For this review, take the finished solid that the model builds, in its own axes (mm). Face numbers are marked on the shaded views. A direction names the side the tool comes from. Coordinates: 2 decimals unless noted, no trailing zeros. Write each loop counter-clockwise with the first axis right and the second up, starting at its lowest first coordinate (ties: lowest second). Pieces come first, ordered by that corner, then holes. Notation, with made-up numbers: (32.25, 77.25) -> (45.25, 77.25) arc R19 ccw to (45.25, 81.25) -> close; hole circle Ø6 at (69.25, -4.5). An arc over 180 degrees is marked (long way). One line per item, written item: value. Start each with the question number.
1) Add section C-C (x = 8.75). State the section outline as (y, z) points.
2) Add section D-D (x = 4.5). State the section outline as (y, z) points, and give its area (3 significant figures).
3) For pin 1 Ø1.5 at (x, y) = (12.5, 31.5) entering from +Z; pin 2 Ø5.5 at (x, z) = (11.5, -1.5) entering from +Y; pin 3 Ø1 at (x, y) = (15, 2) entering from -Z, all flat-tipped, find the tip position at first contact; note any pin that passes through.
4) Add section A-A (x = 17.5). State the section outline as (y, z) points, and give its area (3 significant figures).
5) For probe 1 along Y at (x, z) = (10, -32.75); probe 2 along X at (y, z) = (34, -2.5); probe 3 along Y at (x, z) = (10.75, -31), list the stretches that pass through material, from the lowest coordinate up. Write a range as from..to.
6) Add section B-B (y = 4.5). State the section outline as (x, z) points.
7) Machinability: for the marked faces 1, 2 and 3, which of the approach directions +Z, -Z, +X, -X, +Y, -Y give a long, thin tool a straight path to every point of the face, cutting with its end or side? Answer none if there is none.
from build123d import *

# Parameters (mm, degrees)
SKETCH1_W           = 20
SKETCH1_H           = 46
BOSS_EXTRUDE1_DEPTH = 35
SKETCH2_W           = 5
SKETCH2_H           = 8
CUT_EXTRUDE1_DEPTH  = 5
FILLET1_R           = 2.5
FILLET2_R           = 1
FILLET3_R           = 1
SKETCH3_R           = 9
SKETCH3_R_2         = 6.5
CUT_EXTRUDE2_DEPTH  = 5
FILLET4_R           = 2
FILLET5_R           = 1


with BuildPart() as part:
    # Sketch1 → Boss-Extrude1 (new body)
    with BuildSketch(Plane.XY):
        with Locations((10, 23)):
            Rectangle(SKETCH1_W, SKETCH1_H)
    extrude(amount=-BOSS_EXTRUDE1_DEPTH)

    # Sketch2 → Cut-Extrude1 (cut)
    with BuildSketch(Plane.XY):
        Polygon((10, 41), (2, 41), (2, 46), (20, 46), (20, 41), align=None)
        with Locations((12.5, 32)):
            Rectangle(SKETCH2_W, SKETCH2_H)
    extrude(amount=-CUT_EXTRUDE1_DEPTH, mode=Mode.SUBTRACT)

    # Fillet1
    fillet1_edges = [part.edges().sort_by_distance(p)[0] for p in [
        (11, 41, -5),
    ]]
    fillet(fillet1_edges, radius=FILLET1_R)

    # Fillet2
    fillet2_edges = [part.edges().sort_by_distance(p)[0] for p in [
        (1, 46, 0),
    ]]
    fillet(fillet2_edges, radius=FILLET2_R)

    # Fillet3
    fillet3_edges = [part.edges().sort_by_distance(p)[0] for p in [
        (11, 46, -5),
        (11, 41, 0),
    ]]
    fillet(fillet3_edges, radius=FILLET3_R)

    # Sketch3 → Cut-Extrude2 (cut)
    with BuildSketch(Plane(origin=(0, 0, -35), x_dir=(-1, 0, 0), z_dir=(0, 0, -1))):
        with Locations((-10, 36)):
            Circle(SKETCH3_R)
        with Locations((-10, 36)):
            Circle(SKETCH3_R_2, mode=Mode.SUBTRACT)
        Polygon((-10, 5), (-20, 5), (-20, 0), (-5, 0), (-5, 5), align=None)
    extrude(amount=-CUT_EXTRUDE2_DEPTH, mode=Mode.SUBTRACT)

    # Fillet4
    fillet4_edges = [part.edges().sort_by_distance(p)[0] for p in [
        (12.5, 5, -30),
    ]]
    fillet(fillet4_edges, radius=FILLET4_R)

    # Fillet5
    fillet5_edges = [part.edges().sort_by_distance(p)[0] for p in [
        (12.5, 0, -30),
        (12.5, 5, -35),
        (2.5, 0, -35),
    ]]
    fillet(fillet5_edges, radius=FILLET5_R)


solid = part.part
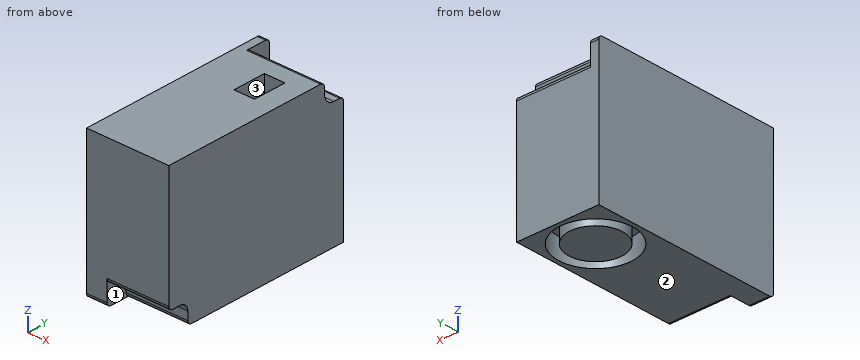
Numbers:
1. outline: (0, -29) arc R1 ccw to (1, -30) -> (3, -30) arc R2 cw to (5, -32) -> (5, -34) arc R1 ccw to (6, -35) -> (27.09, -35) -> (27.09, -30) -> (29.62, -30) -> (29.62, -35) -> (42.38, -35) -> (42.38, -30) -> (44.91, -30) -> (44.91, -35) -> (46, -35) -> (46, -6) arc R1 ccw to (45, -5) -> (43.5, -5) arc R2.5 cw to (41, -2.5) -> (41, -1) arc R1 ccw to (40, 0) -> (0, 0) -> close
2. outline: (0, -34) arc R1 ccw to (1, -35) -> (28.88, -35) -> (28.88, -30) -> (32.54, -30) -> (32.54, -35) -> (39.46, -35) -> (39.46, -30) -> (43.12, -30) -> (43.12, -35) -> (46, -35) -> (46, -6) arc R1 ccw to (45, -5) -> (43.5, -5) arc R2.5 cw to (41, -2.5) -> (41, -1) arc R1 ccw to (40, 0) -> (0, 0) -> close
2. area: 1,550 mm²
3. pin 1: z = -5
3. pin 2: y = 41.71
3. pin 3: z = -30
4. outline: (0, -29) arc R1 ccw to (1, -30) -> (3, -30) arc R2 cw to (5, -32) -> (5, -34) arc R1 ccw to (6, -35) -> (31.03, -35) -> (31.03, -30) -> (40.97, -30) -> (40.97, -35) -> (46, -35) -> (46, -6) arc R1 ccw to (45, -5) -> (43.5, -5) arc R2.5 cw to (41, -2.5) -> (41, -1) arc R1 ccw to (40, 0) -> (0, 0) -> close
4. area: 1,510 mm²
5. probe 1: 5..27, 29.5..42.5, 45..46
5. probe 2: 0..10, 15..20
5. probe 3: 4.73..27.03, 29.54..42.46, 44.97..46
6. outline: (0, -35) -> (5, -35) -> (5, -30.68) -> (20, -30.68) -> (20, 0) -> (0, 0) -> close
7. face 1: -Z, +X, -Y
7. face 2: -Z, +X, -X, +Y, -Y
7. face 3: +Z
